Input: part model. Units: mm. Frame: model coordinates. A direction names the side the tool comes from. Give positions to 0.01 mm unless a question says otherwise; leave off trailing zeros. One line per question, with ' | ' between items.
from build123d import *

# Parameters (mm, degrees)
SKETCH6_W                     = 2.15
SKETCH6_H                     = 89.5
M4_CLEARANCE_HOLE2_AT_2_COUNT = 2
M4_CLEARANCE_HOLE2_AT_2_PITCH = 11
M4_CLEARANCE_HOLE2_AT_3_COUNT = 2
M4_CLEARANCE_HOLE2_AT_3_PITCH = 19.052558883
M4_CLEARANCE_HOLE2_AT_4_COUNT = 2
M4_CLEARANCE_HOLE2_AT_4_PITCH = 22
M4_CLEARANCE_HOLE2_AT_5_COUNT = 2
M4_CLEARANCE_HOLE2_AT_5_PITCH = 19.052558883
M4_CLEARANCE_HOLE2_AT_6_COUNT = 2
M4_CLEARANCE_HOLE2_AT_6_PITCH = 11
M4_TAPPED_HOLE1_AT_2_COUNT    = 2
M4_TAPPED_HOLE1_AT_2_PITCH    = 11
M4_TAPPED_HOLE1_AT_3_COUNT    = 2
M4_TAPPED_HOLE1_AT_3_PITCH    = 19.052558883
M4_TAPPED_HOLE1_AT_4_COUNT    = 2
M4_TAPPED_HOLE1_AT_4_PITCH    = 11
M4_TAPPED_HOLE1_AT_5_COUNT    = 2
M4_TAPPED_HOLE1_AT_5_PITCH    = 19.052558883
M4_TAPPED_HOLE1_AT_6_COUNT    = 2
M4_TAPPED_HOLE1_AT_6_PITCH    = 22
M5_TAPPED_HOLE1_AT_2_COUNT    = 2
M5_TAPPED_HOLE1_AT_2_PITCH    = 18.03122292
M5_TAPPED_HOLE1_AT_3_COUNT    = 2
M5_TAPPED_HOLE1_AT_3_PITCH    = 19.596880573
M5_TAPPED_HOLE1_AT_4_COUNT    = 2
M5_TAPPED_HOLE1_AT_4_PITCH    = 25.394250395
CHAMFER1_SIZE                 = 0.6
FILLET1_R                     = 0.3
CHAMFER2_SIZE                 = 0.5
FILLET2_R                     = 0.4
FILLET3_R                     = 0.4


with BuildPart() as part:
    # Sketch1 → Revolve1 (revolve)
    with BuildSketch(Plane(origin=(0, 0, 0), x_dir=(0, 0, -1), z_dir=(1, 0, 0)), mode=Mode.PRIVATE) as revolve1_sk:
        Polygon((55, 102.5), (55, 92.5), (54.5, 92.5), (54.5, 36.5), (55, 36.5), (55, 27.5), (57, 27.5), (57, 20.5), (57, 16.5), (48.5, 16.5), (48.5, 14.5), (47, 14.5), (47, 102.5), align=None)
    revolve(revolve1_sk.sketch.rotate(Axis((0, 110.959510929, -40), (0, -1, 0)), 180), axis=Axis((0, 110.959510929, -40), (0, -1, 0)))

    # Sketch12 → M4 Tapped Hole1 (revolve, cut)
    with BuildSketch(Plane(origin=(0, 102.5, -51), x_dir=(0, 0, 1), z_dir=(1, 0, 0))):
        Polygon((0, 0), (0, 12.491420021), (1.65, 11.5), (1.65, 0), align=None)
    m4_tapped_hole1 = revolve(axis=Axis((0, 108.85, -51), (0, -1, 0)), mode=Mode.SUBTRACT)

    # M4 Tapped Hole1 at 2: M4 Tapped Hole1 ×2
    with Locations(*[Vector(0.8660254037844388, 0, 0.49999999999999983) * (i * M4_TAPPED_HOLE1_AT_2_PITCH) for i in range(1, M4_TAPPED_HOLE1_AT_2_COUNT)]):
        add(m4_tapped_hole1, mode=Mode.SUBTRACT)

    # M4 Tapped Hole1 at 3: M4 Tapped Hole1 ×2
    with Locations(*[Vector(0.5000000000000001, 0, 0.8660254037844386) * (i * M4_TAPPED_HOLE1_AT_3_PITCH) for i in range(1, M4_TAPPED_HOLE1_AT_3_COUNT)]):
        add(m4_tapped_hole1, mode=Mode.SUBTRACT)

    # M4 Tapped Hole1 at 4: M4 Tapped Hole1 ×2
    with Locations(*[Vector(-0.8660254037844386, 0, 0.5000000000000003) * (i * M4_TAPPED_HOLE1_AT_4_PITCH) for i in range(1, M4_TAPPED_HOLE1_AT_4_COUNT)]):
        add(m4_tapped_hole1, mode=Mode.SUBTRACT)

    # M4 Tapped Hole1 at 5: M4 Tapped Hole1 ×2
    with Locations(*[Vector(-0.4999999999999999, 0, 0.8660254037844388) * (i * M4_TAPPED_HOLE1_AT_5_PITCH) for i in range(1, M4_TAPPED_HOLE1_AT_5_COUNT)]):
        add(m4_tapped_hole1, mode=Mode.SUBTRACT)

    # M4 Tapped Hole1 at 6: M4 Tapped Hole1 ×2
    with Locations(*[(0, 0, i * M4_TAPPED_HOLE1_AT_6_PITCH) for i in range(1, M4_TAPPED_HOLE1_AT_6_COUNT)]):
        add(m4_tapped_hole1, mode=Mode.SUBTRACT)

    # Sketch15 → M5 Tapped Hole1 (revolve, cut)
    with BuildSketch(Plane(origin=(9.01561146, 16.5, -49.01561146), x_dir=(0, 0, -1), z_dir=(1, 0, 0))):
        Polygon((0, 0), (0, 11.2618073), (2.1, 10), (2.1, 0), align=None)
    m5_tapped_hole1 = revolve(axis=Axis((9.01561146, 10.15, -49.01561146), (0, 1, 0)), mode=Mode.SUBTRACT)

    # M5 Tapped Hole1 at 2: M5 Tapped Hole1 ×2
    with Locations(*[(-i * M5_TAPPED_HOLE1_AT_2_PITCH, 0, 0) for i in range(1, M5_TAPPED_HOLE1_AT_2_COUNT)]):
        add(m5_tapped_hole1, mode=Mode.SUBTRACT)

    # M5 Tapped Hole1 at 3: M5 Tapped Hole1 ×2
    with Locations(*[Vector(-0.09097740748886197, 0, 0.9958529566791503) * (i * M5_TAPPED_HOLE1_AT_3_PITCH) for i in range(1, M5_TAPPED_HOLE1_AT_3_COUNT)]):
        add(m5_tapped_hole1, mode=Mode.SUBTRACT)

    # M5 Tapped Hole1 at 4: M5 Tapped Hole1 ×2
    with Locations(*[Vector(-0.639843636962356, 0, 0.768505120502645) * (i * M5_TAPPED_HOLE1_AT_4_PITCH) for i in range(1, M5_TAPPED_HOLE1_AT_4_COUNT)]):
        add(m5_tapped_hole1, mode=Mode.SUBTRACT)

    # Chamfer1
    chamfer1_edges = [part.edges().sort_by_distance(p)[0] for p in [
        (0, 102.5, -55),
    ]]
    chamfer(chamfer1_edges, length=CHAMFER1_SIZE)

    # Fillet1
    fillet1_edges = [part.edges().sort_by_distance(p)[0] for p in [
        (0, 27.5, -55),
    ]]
    fillet(fillet1_edges, radius=FILLET1_R)

    # Chamfer2
    chamfer2_edges = [part.edges().sort_by_distance(p)[0] for p in [
        (0, 92.5, -54.5),
        (0, 36.5, -54.5),
    ]]
    chamfer(chamfer2_edges, length=CHAMFER2_SIZE - 0.0001)  # a hair under: the kernel refuses the full size

    # Fillet2
    fillet2_edges = [part.edges().sort_by_distance(p)[0] for p in [
        (0, 16.5, -48.5),
    ]]
    fillet(fillet2_edges, radius=FILLET2_R)


with BuildPart() as body_2:
    # Sketch2 → Revolve2 (revolve)
    with BuildSketch(Plane(origin=(0, 0, 0), x_dir=(0, 0, -1), z_dir=(1, 0, 0)), mode=Mode.PRIVATE) as revolve2_sk:
        Polygon((47, 106), (57, 106), (57, 101.5), (55, 101.5), (55, 103), (47, 103), align=None)
    revolve(revolve2_sk.sketch.rotate(Axis((0, 110.959510929, -40), (0, -1, 0)), 180), axis=Axis((0, 110.959510929, -40), (0, -1, 0)))

    # Sketch6 → M4 Clearance Hole2 (revolve, cut)
    with BuildSketch(Plane(origin=(-9.526279442, 106, -45.5), x_dir=(0, 0, 1), z_dir=(1, 0, 0))):
        with Locations((1.075, 44.75)):
            Rectangle(SKETCH6_W, SKETCH6_H)
    m4_clearance_hole2 = revolve(axis=Axis((-9.526279442, 112.35, -45.5), (0, -1, 0)), mode=Mode.SUBTRACT)

    # M4 Clearance Hole2 at 2: M4 Clearance Hole2 ×2
    with Locations(*[Vector(0.8660254037844386, 0, -0.5000000000000003) * (i * M4_CLEARANCE_HOLE2_AT_2_PITCH) for i in range(1, M4_CLEARANCE_HOLE2_AT_2_COUNT)]):
        add(m4_clearance_hole2, mode=Mode.SUBTRACT)

    # M4 Clearance Hole2 at 3: M4 Clearance Hole2 ×2
    with Locations(*[(i * M4_CLEARANCE_HOLE2_AT_3_PITCH, 0, 0) for i in range(1, M4_CLEARANCE_HOLE2_AT_3_COUNT)]):
        add(m4_clearance_hole2, mode=Mode.SUBTRACT)

    # M4 Clearance Hole2 at 4: M4 Clearance Hole2 ×2
    with Locations(*[Vector(0.8660254037844387, 0, 0.49999999999999994) * (i * M4_CLEARANCE_HOLE2_AT_4_PITCH) for i in range(1, M4_CLEARANCE_HOLE2_AT_4_COUNT)]):
        add(m4_clearance_hole2, mode=Mode.SUBTRACT)

    # M4 Clearance Hole2 at 5: M4 Clearance Hole2 ×2
    with Locations(*[Vector(0.5000000000000001, 0, 0.8660254037844387) * (i * M4_CLEARANCE_HOLE2_AT_5_PITCH) for i in range(1, M4_CLEARANCE_HOLE2_AT_5_COUNT)]):
        add(m4_clearance_hole2, mode=Mode.SUBTRACT)

    # M4 Clearance Hole2 at 6: M4 Clearance Hole2 ×2
    with Locations(*[(0, 0, i * M4_CLEARANCE_HOLE2_AT_6_PITCH) for i in range(1, M4_CLEARANCE_HOLE2_AT_6_COUNT)]):
        add(m4_clearance_hole2, mode=Mode.SUBTRACT)

    # Fillet3
    fillet3_edges = [body_2.edges().sort_by_distance(p)[0] for p in [
        (0, 103, -55),
    ]]
    fillet(fillet3_edges, radius=FILLET3_R)


solid = part.part
1. Reachability of faces 1 (the cylindrical face through (8.385, 21.43, -51.019)), 2 (the cylindrical face through (-8.06, 96.83, -33.74)) from +Z, -Z, +X, -X, +Y, -Y: full face, straight path, thin tool, end or side. Return the list, or none.
Determined:
face 1: -Y | face 2: +Y
2. Pin query (flat end, axial travel): P1, Ø5, axis at x = -9.02, z = -49.02, coming from the -Y side; P2, Ø3, axis at x = 9.53, z = -34.5, coming from the +Y side; P3, Ø1.5, axis at x = 8.5, z = -41.5, coming from the -Y side; P4, Ø2, axis at y = 67.5, z = -51, coming from the +X side. Return the tip coordinate at first contact, or that it passes through.
Determined:
P1: stops at y = 16.5 | P2: stops at y = 90.91 | P3: stops at y = 14.5 | P4: stops at x = 10.5
3. Ray query, line 1 along X through (y, z) = (36, -39.5); line 2 along X through (y, z) = (93, -45); line 3 along X through (y, z) = (67, -40). Return the intervals inside material, ascending. Write a range as from..to.
Determined:
line 1: x = -14.99..-6.98, 6.98..14.99 | line 2: x = -14.14..-11.1, -7.95..-4.9, 4.9..7.95, 11.1..14.14 | line 3: x = -14.5..-7, 7..14.5
